The listing builds one solid part. Answer for the finished solid, in the listing's coordinates (mm). Face numbers are marked on the shaded views. A direction names the side the tool comes from. Round coordinates to 2 decimals unless told otherwise and drop trailing zeros. Write each loop counter-clockwise with the first axis right and the second up, starting at its lowest first coordinate (ties: lowest second). Pieces come first, ordered by that corner, then holes. Notation, with made-up numbers: M -21.5,81 L 19.5,81 A27 cw 19.5,97 Z; hole C 39,-20 d1. An arc over 180 degrees is marked long. One line per item, written item: value. Start each with the question number.
(1) Section C-C (z = 14.5) is taken. Determine the outline of the cut face in (x, y).
(2) Section A-A (z = 18) is taken. Determine the outline of the cut face in (x, y), plus the area to 3 significant figures.
(3) For a pull along Y with two mould halves and no side action, classify the marked faces 3, 4 and 5 as released by +Y, released by -Y, zero draft, split by the parting line, or undercut.
(4) Consider probe 1 along Y at (x, z) = (-19, 38.5); probe 2 along X at (y, z) = (1, 16); probe 3 along Y at (x, z) = (-32.75, 24). Determine where each line is inside the solid, lowest interval first.
(5) For the marked faces 1 and 2, determine the directions among +Z, -Z, +X, -X, +Y, -Y from which every point of the face is accessible in a straight line to the end or side of a thin tool.
(6) Given P1, Ø2.5, axis at x = -21.2, z = 37.63, coming from the +Y side, flat-ended and moving along its own axis, determine where the tip first touches the part or whether it passes through.
(7) Section B-B (x = -27.75) is taken. Determine the outline of the cut face in (y, z).
(8) Section D-D (x = -20) is taken. State how many separate pieces and enclosed holes the cut face has, plus the area to 3 significant figures.
```python
from build123d import *

# Parameters (mm, degrees)
F0_W          = 25
F0_H          = 30
F0_R          = 2.1
F1_DEPTH      = 2
F2_W          = 25
F2_H          = 2
F2_H_2        = 4.2
F3_DEPTH      = 2
F4_DEPTH      = 30
F5_R          = 2.1
F6_DEPTH      = 8.2
F8_R          = 8.1
F8_R_2        = 2.1
F9_DEPTH      = 2.5
F9_DEPTH_BACK = 3.5
F10_R         = 4.1
F11_DEPTH     = 1
F12_R         = 2
F13_DEPTH     = 8.2


with BuildPart() as f1:
    # F0 (on Front) → F1 (new body)
    with BuildSketch(Plane.XZ):
        with Locations((-27.446082, 26.626395)):
            Rectangle(F0_W, F0_H)
        with Locations((-27.446082, 26.626395)):
            Circle(F0_R, mode=Mode.SUBTRACT)
    extrude(amount=-F1_DEPTH)

    # F2 (on face) → F3 (join)
    with BuildSketch(Plane.XY.offset(41.626395)):
        with Locations((-27.446082, 7.2)):
            Rectangle(F2_W, F2_H)
        with Locations((-27.446082, 4.1)):
            Rectangle(F2_W, F2_H_2)
        with Locations((-27.446082, 1)):
            Rectangle(F2_W, F2_H)
    extrude(amount=F3_DEPTH)

    # F2 (on face) → F4 (join)
    with BuildSketch(Plane.XY.offset(41.626395)):
        with Locations((-27.446082, 7.2)):
            Rectangle(F2_W, F2_H)
    extrude(amount=-F4_DEPTH)

    # F5 (on face) → F6 (cut, through all)
    with BuildSketch(Plane.XZ):
        with Locations((-27.446082, 26.626395)):
            Circle(F5_R)
    extrude(amount=-F6_DEPTH, mode=Mode.SUBTRACT)

    # F8 (on offset) → F9 (cut, two sides)
    with BuildSketch(Plane.XZ.offset(-3.5)) as f9_sk:
        with Locations((-27.446082, 26.626395)):
            Circle(F8_R)
        with Locations((-27.446082, 26.626395)):
            Circle(F8_R_2, mode=Mode.SUBTRACT)
    extrude(amount=F9_DEPTH, mode=Mode.SUBTRACT)
    extrude(f9_sk.sketch, amount=-F9_DEPTH_BACK, mode=Mode.SUBTRACT)

    # F10 (on face) → F11 (cut, through all)
    with BuildSketch(Plane.XZ):
        with Locations((-27.446082, 26.626395)):
            Circle(F10_R)
    extrude(amount=-F11_DEPTH, mode=Mode.SUBTRACT)

    # F12 (on face) → F13 (cut, through all)
    with BuildSketch(Plane(origin=(0, 8.2, 0), x_dir=(-1, 0, 0), z_dir=(0, 1, 0))):
        with Locations((21.196082, 37.626395)):
            Circle(F12_R)
        with Locations((33.696082, 37.626395)):
            Circle(F12_R)
        with Locations((21.196082, 15.626395)):
            Circle(F12_R)
        with Locations((33.696082, 15.626395)):
            Circle(F12_R)
    extrude(amount=-F13_DEPTH, mode=Mode.SUBTRACT)


solid = f1.part
```
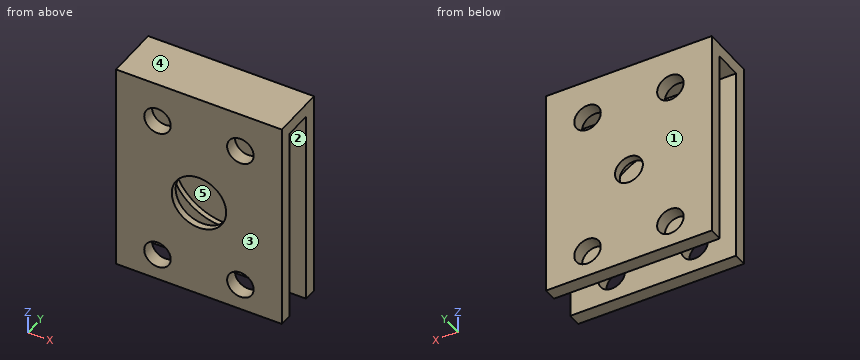
Recorded:
1. outline: M -39.95,0 L -35.35,0 L -35.35,2 L -39.95,2 Z; M -39.95,6.2 L -35.35,6.2 L -35.35,8.2 L -39.95,8.2 Z; M -32.04,0 L -22.85,0 L -22.85,2 L -32.04,2 Z; M -32.04,6.2 L -22.85,6.2 L -22.85,8.2 L -32.04,8.2 Z; M -19.54,0 L -14.95,0 L -14.95,2 L -19.54,2 Z; M -19.54,6.2 L -14.95,6.2 L -14.95,8.2 L -19.54,8.2 Z
2. outline: M -39.95,0 L -14.95,0 L -14.95,2 L -39.95,2 Z; M -39.95,6.2 L -14.95,6.2 L -14.95,8.2 L -39.95,8.2 Z
2. area: 100 mm2
3. face 3: released by -Y
3. face 4: zero draft
3. face 5: undercut
4. probe 1: y = 0 to 2, 6.2 to 8.2
4. probe 2: x = -39.95 to -35.66, -31.73 to -23.16, -19.23 to -14.95
4. probe 3: y = 0 to 1, 7 to 8.2
5. face 1: +Z, -Z, +X, -X, +Y
5. face 2: -Z, +X, -X
6. P1: passes through
7. outline: M 0,11.63 L 2,11.63 L 2,18.53 L 1,18.53 L 1,22.54 L 0,22.54 Z; M 0,30.72 L 1,30.72 L 1,34.72 L 2,34.72 L 2,41.63 L 6.2,41.63 L 6.2,34.72 L 7,34.72 L 7,28.7 L 8.2,28.7 L 8.2,43.63 L 0,43.63 Z; M 6.2,11.63 L 8.2,11.63 L 8.2,24.55 L 7,24.55 L 7,18.53 L 6.2,18.53 Z
8. separate pieces: 5
8. enclosed holes: 0
8. area: 99.3 mm2
